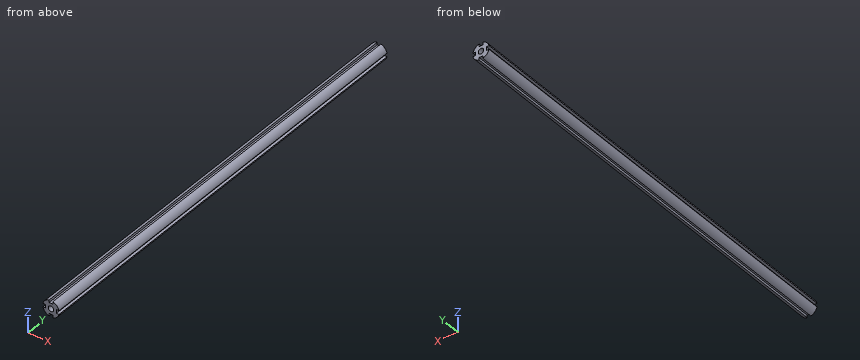
```python
from build123d import *

# Parameters (mm, degrees)
SKETCH1_R                 = 4.5
BOSS_EXTRUDE1_DEPTH       = 232
F_3_0MM_DOWEL_HOLE1_D     = 3
F_3_0MM_DOWEL_HOLE1_DEPTH = 3
F_3_0MM_DOWEL_HOLE1_TIP   = 0.901290929
F_3_0MM_DOWEL_HOLE2_D     = 3
F_3_0MM_DOWEL_HOLE2_DEPTH = 3
F_3_0MM_DOWEL_HOLE2_TIP   = 0.901290929
SKETCH6_W                 = 2
SKETCH6_H                 = 2
CUT_EXTRUDE1_DEPTH        = 233.08726807
CIRPATTERN1_COUNT         = 4


with BuildPart() as part:
    # Sketch1 → Boss-Extrude1 (new body)
    with BuildSketch(Plane(origin=(0, 0, 0), x_dir=(1, 0, 0), z_dir=(0, 1, 0))):
        with Locations(Location((0, 0, 0), (0, 0, 90))):
            Circle(SKETCH1_R)
    extrude(amount=BOSS_EXTRUDE1_DEPTH)

    # Ø3.0mm Dowel Hole1
    with Locations(Plane.XZ):
        with Locations((0, 0)):
            Hole(F_3_0MM_DOWEL_HOLE1_D / 2, depth=F_3_0MM_DOWEL_HOLE1_DEPTH)
            with Locations((0, 0, -(F_3_0MM_DOWEL_HOLE1_DEPTH + F_3_0MM_DOWEL_HOLE1_TIP / 2))):  # 118° drill point
                Cone(0, F_3_0MM_DOWEL_HOLE1_D / 2, F_3_0MM_DOWEL_HOLE1_TIP, mode=Mode.SUBTRACT)

    # Ø3.0mm Dowel Hole2
    with Locations(Plane(origin=(0, 232, 0), x_dir=(1, 0, 0), z_dir=(0, 1, 0))):
        with Locations((0, 0)):
            Hole(F_3_0MM_DOWEL_HOLE2_D / 2, depth=F_3_0MM_DOWEL_HOLE2_DEPTH)
            with Locations((0, 0, -(F_3_0MM_DOWEL_HOLE2_DEPTH + F_3_0MM_DOWEL_HOLE2_TIP / 2))):  # 118° drill point
                Cone(0, F_3_0MM_DOWEL_HOLE2_D / 2, F_3_0MM_DOWEL_HOLE2_TIP, mode=Mode.SUBTRACT)

    # Sketch6 → Cut-Extrude1 (cut, through all)
    with BuildSketch(Plane(origin=(0, 232, 0), x_dir=(1, 0, 0), z_dir=(0, 1, 0))):
        with Locations((-4, 0)):
            Rectangle(SKETCH6_W, SKETCH6_H)
    cut_extrude1 = extrude(amount=-CUT_EXTRUDE1_DEPTH, mode=Mode.SUBTRACT)

    # CirPattern1: Cut-Extrude1 ×4 about axis
    cirpattern1_axis = Axis((0, 0, 0), (0, 1, 0))
    for i in range(1, CIRPATTERN1_COUNT):
        add(cut_extrude1.rotate(cirpattern1_axis, i * 360 / CIRPATTERN1_COUNT), mode=Mode.SUBTRACT)


solid = part.part
```
The listing builds one solid part. Answer for the finished solid, in the listing's coordinates (mm). Give positions to 0.01 mm unless a question says otherwise; leave off trailing zeros. Order: outer loops, then holes, each group sorted by start corner. A loop starts at its lowest first (then second) coordinate and runs counter-clockwise, first axis right, second up. Notation, with made-up numbers: (81.5, -4.75) -> (135.5, -4.75) arc R22 ccw to (135.5, 28.25) -> close; hole circle Ø8 at (82.5, -14). An arc over 180 degrees is marked (long way). Answer as CSV lines item,"result". Start each with the question number.
Q1. Given pin 1 (2 mm diameter, centred on y = 77, z = 0.5, fed in from +X); pin 2 (1.6 mm diameter, centred on y = 87, z = 0, fed in from -X); pin 3 (2.5 mm diameter, centred on x = 0, z = 0, fed in from -Y); pin 4 (0.7 mm diameter, centred on x = 3.5, y = 156, fed in from +Z), each flat-ended and moving along its own axis, determine where each tip first touches the part or whether it passes through.
Q2. Find the intervals of material crossed by L1, parallel to Z at x = 0, y = 230.65; L2, parallel to Z at x = -0.25, y = 217.5, in increasing order.
Q3. A cutting plane is placed at A-A (y = 104). Determine the outline of the cut face in (x, z), then the cut area to 3 significant figures.
Results found:
1,pin 1,"x = 4.39"
1,pin 2,"x = -3"
1,pin 3,"y = 3.15"
1,pin 4,"z = 3.21"
2,L1,"-3 to -1.5, 1.5 to 3"
2,L2,"-3 to 3"
3,outline,"(-4.39, -1) arc R4.5 ccw to (-1, -4.39) -> (-1, -3) -> (1, -3) -> (1, -4.39) arc R4.5 ccw to (4.39, -1) -> (3, -1) -> (3, 1) -> (4.39, 1) arc R4.5 ccw to (1, 4.39) -> (1, 3) -> (-1, 3) -> (-1, 4.39) arc R4.5 ccw to (-4.39, 1) -> (-3, 1) -> (-3, -1) -> close"
3,area,"51.9 mm2"
